Geometry: final body of the model. Coordinates: model frame, mm. A direction names the side the tool comes from. Coordinates: 2 decimals unless noted, no trailing zeros. Order: outer loops, then holes, each group sorted by start corner. A loop starts at its lowest first (then second) coordinate and runs counter-clockwise, first axis right, second up. Notation, with made-up numbers: M 43.25,-25.5 L 86.25,-25.5 A20 cw 86.25,-17.5 Z; hole C 69,56 d2. An arc over 180 degrees is marked long. Use CSV: the item, a comma, the result in double quotes. Start each with the question number.
Q1. First-contact query: P1, Ø3, axis at y = 48, z = -4, coming from the +X side. Flat tip, straight axial feed; report the tip coordinate or a pass-through.
Q2. Ray query, probe 1 along Z at (x, y) = (-2.4, 27.5); probe 2 along Y at (x, z) = (-3.6, -3); probe 3 along Z at (x, y) = (-4.8, 47.5). Return the intervals inside material, ascending.
Q3. Access query for faces 1 (the face through (-3.5, 29, -6)), 2 (the face through (-5.5, 27.1, -6.4)). Directions: +Z, -Z, +X, -X, +Y, -Y. A direction counts if a zero-diameter tool reaches every point of the face in a straight line with its end or side. Return the directions, or none.
Q4. Mould query, pull axis Z, two halves, no side actions, for faces 3 (the face through (-3, 0, -4)), 4 (the face through (-3, 27, 0)), 5 (the face through (-3, 27, -9)), 6 (the face through (-4.51, 8.56, -3.11)). Classes: +Z half, -Z half, draft (parallel to the pull), parting line (faces both ways), or undercut.
Q5. Section query A-A, the plane y = 47.5. Output: boundary loops of the cut face in (x, z), and give its area (3 significant figures).
Q6. Section query C-C, the plane x = -0.55. Output: boundary loops of the cut face in (y, z).
Q7. Section query B-B, the plane z = -4.5. Output: boundary loops of the cut face in (x, y).
Autodesk Inventor part; units mm, degrees
ref_plane "YZ Plane" through (0, 0, 0) normal (1, 0, 0) x (0, 1, 0)
ref_plane "XZ Plane" through (0, 0, 0) normal (0, 1, 0) x (-1, 0, 0)
ref_plane "XY Plane" through (0, 0, 0) normal (0, 0, 1) x (1, 0, 0)
sketch "スケッチ1" plane through (0, 0, 0) normal (0, 1, 0) x (-1, 0, 0)
  line L0 (0, 0) -> (5.5, 0)
  line L1 (5.5, 0) -> (5.5, -9)
  line L2 (5.5, -9) -> (0, -9)
  line L3 (0, -9) -> (0, 0)
  dimension "d0" = 5.5
  dimension "d1" = 9
extrude "押し出し1" add sketch "スケッチ1" along normal blind 55
sketch "スケッチ2" plane through (0, 0, 0) normal (1, 0, 0) x (0, 0, -1)
  line L0 (0, 55) -> (9, 55)
  line L1 (4.5, 55) -> (4.5, 0)
  line L2 (9, 0) -> (0, 0)
  point P0 (4.5, 27.5)
  point P1 (4.5, 47.5)
  point P2 (4.5, 7.5)
  dimension "d4" = 27.5
  dimension "d5" = 20
  dimension "d6" = 20
hole "穴1" at (0, 27.5, -4.5) at (0, 47.5, -4.5) at (0, 7.5, -4.5) direction (-1, 0, 0) diameter 3.5 depth 8 tip angle 118 counterbore diameter 6 counterbore depth 3.5
properties part number "rail_SSEB10"
Responses:
1,P1,"stops at x = -3.5"
2,probe 1,"z = -9 to -7.5, -1.5 to 0"
2,probe 2,"y = 0 to 6.6, 8.4 to 26.6, 28.4 to 46.6, 48.4 to 55"
2,probe 3,"z = -9 to -6.25, -2.75 to 0"
3,face 1,"+X"
3,face 2,"+Z, -Z, -X, +Y, -Y"
4,face 3,"draft"
4,face 4,"+Z half"
4,face 5,"-Z half"
4,face 6,"undercut"
5,outline,"M -5.5,-9 L 0,-9 L 0,-7.5 L -3.5,-7.5 L -3.5,-6.25 L -5.5,-6.25 Z; M -5.5,-2.75 L -3.5,-2.75 L -3.5,-1.5 L 0,-1.5 L 0,0 L -5.5,0 Z"
5,area,"21.5 mm²"
6,outline,"M 0,-9 L 55,-9 L 55,0 L 0,0 Z; hole C 7.5,-4.5 d6; hole C 27.5,-4.5 d6; hole C 47.5,-4.5 d6"
7,outline,"M -5.5,0 L 0,0 L 0,4.5 L -3.5,4.5 L -3.5,5.75 L -5.5,5.75 Z; M -5.5,9.25 L -3.5,9.25 L -3.5,10.5 L 0,10.5 L 0,24.5 L -3.5,24.5 L -3.5,25.75 L -5.5,25.75 Z; M -5.5,29.25 L -3.5,29.25 L -3.5,30.5 L 0,30.5 L 0,44.5 L -3.5,44.5 L -3.5,45.75 L -5.5,45.75 Z; M -5.5,49.25 L -3.5,49.25 L -3.5,50.5 L 0,50.5 L 0,55 L -5.5,55 Z"
